Design review of the part built by this model. Coordinates are the model's own, in mm. Face numbers are marked on the shaded views. A direction names the side the tool comes from. Round coordinates to 2 decimals unless told otherwise and drop trailing zeros. Write each loop counter-clockwise with the first axis right and the second up, starting at its lowest first coordinate (ties: lowest second). Pieces come first, ordered by that corner, then holes. Notation, with made-up numbers: M -1.75,37.5 L 53.25,37.5 A20 ccw 53.25,54.5 Z; hole C 40.5,-16 d2. An arc over 180 degrees is marked long. Use CSV: the item, a comma, the result in double quotes.
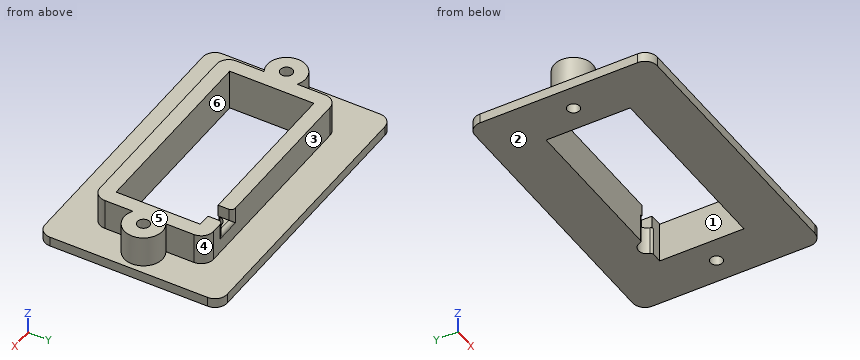
Autodesk Fusion 360 part; units mm, degrees
sketch "Sketch1" plane through (0, 0, 0) normal (0, 0, 1) x (1, 0, 0)
  line L0 (11.6, 5.15) -> (-11.6, 5.15)
  line L1 (-11.6, 5.15) -> (-11.6, -5.15)
  line L2 (-11.6, -5.15) -> (11.6, -5.15)
  line L3 (11.6, -5.15) -> (11.6, 5.15)
  line L4 (11.6, 5.15) -> (-11.6, -5.15) construction
  line L5 (-11.6, 5.15) -> (11.6, -5.15) construction
  line L6 (-17.6, -11.15) -> (17.6, -11.15)
  line L7 (17.6, -11.15) -> (17.6, 11.15)
  line L8 (17.6, 11.15) -> (-17.6, 11.15)
  line L9 (-17.6, 11.15) -> (-17.6, -11.15)
  line L10 (13.4, 6.95) -> (-13.4, 6.95)
  line L11 (-13.4, 6.95) -> (-13.4, -6.95)
  line L12 (-13.4, -6.95) -> (13.4, -6.95)
  line L13 (13.4, -6.95) -> (13.4, 6.95)
  dimension "d1" = 23.2
  dimension "d2" = 10.3
  dimension "d3" = 6
  dimension "d4" = 1.8
extrude "Extrude1" add sketch "Sketch1" along normal blind 7 contours L10 L11 L12 L13
extrude "Extrude2" add sketch "Sketch1" along normal blind 1.2 contours L6 L7 L8 L9
sketch "Sketch2" plane through (0, 0, 0) normal (0, 0, 1) x (1, 0, 0)
  line L0 (-22, 0) -> (23, 0) construction
  circle A0 centre (14.6, 0) radius 0.75 construction
  line L1 (11.6, -5.15) -> (11.6, 5.15) construction
  dimension "d9" = 1.5
  dimension "d10" = 3
sketch "Sketch3" plane through (0, 0, 1.2) normal (0, 0, 1) x (-1, 0, 0)
  line L0 (-13.4, -6.95) -> (-13.4, 6.95)
  line L1 (-13.4, 6.95) -> (13.4, 6.95)
  line L2 (13.4, 6.95) -> (13.4, -6.95)
  line L3 (13.4, -6.95) -> (-13.4, -6.95)
  line L4 (17.6, -11.15) -> (17.6, 11.15)
  line L5 (17.6, 11.15) -> (-17.6, 11.15)
  line L6 (-17.6, 11.15) -> (-17.6, -11.15)
  line L7 (-17.6, -11.15) -> (17.6, -11.15)
  circle A0 centre (-14.6, 0) radius 0.75
  circle A1 centre (-14.6, 0) radius 2.35
  dimension "d11" = 1.6
extrude "Extrude3" add sketch "Sketch3" along normal blind 5 contours L0 A1 picked at (-13.55, 0)
extrude "Extrude9" cut 1 faces at (14.8389, -0.0008, 1.2) along direction (0, 0, -1) up to surface (1.2 mm away)
mirror "Mirror1" about plane through (0, 0, 0) normal (1, 0, 0) of "Extrude2", "Extrude3"
sketch "Sketch4" plane through (0, 0, 0) normal (0, 0, 1) x (1, 0, 0)
  line L0 (11.6, -1) -> (17.6, -1)
  line L1 (17.6, -1) -> (17.6, 0.9)
  line L2 (17.6, 0.9) -> (11.6, 0.9)
  line L3 (11.6, 0.9) -> (11.6, -1)
sketch "Sketch5" plane through (0, 0, 0) normal (0, 0, 1) x (1, 0, 0)
  arc A0 (10.0479, 5.1477) -> (7.9479, 5.146) centre (8.9979, 5.148) ccw
  line L0 (7.9479, 5.146) -> (10.0479, 5.1477)
  dimension "d17" = 1.05
extrude "Extrude4" cut sketch "Sketch5" along normal up to surface (7 mm away)
extrude "Extrude5" add 2 faces at (13.55, 0, 6.2) (-13.55, 0, 6.2) along direction (0, 0, 1) up to surface end surface through (0, 0, 7) normal (0, 0, 1) offset 0
sketch "Sketch6" plane through (0, 0, 7) normal (0, 0, 1) x (-1, 0, 0)
  circle A0 centre (14.6, 0) radius 0.75
  circle A1 centre (-14.6, 0) radius 0.75
  line L0 (-13.4, 6.95) -> (-13.4, 2.0205)
  arc A2 (-13.4, 2.0205) -> (-13.4, -2.0205) centre (-14.6, 0) ccw
  line L1 (-13.4, -2.0205) -> (-13.4, -6.95)
  line L2 (-13.4, -6.95) -> (13.4, -6.95)
  line L3 (13.4, -6.95) -> (13.4, -2.0205)
  arc A3 (13.4, -2.0205) -> (13.4, 2.0205) centre (14.6, 0) ccw
  line L4 (13.4, 2.0205) -> (13.4, 6.95)
  line L5 (13.4, 6.95) -> (-13.4, 6.95)
  arc A4 (-10.0479, -5.15) -> (-7.9479, -5.15) centre (-8.9979, -5.148) ccw
  line L6 (-10.0479, -5.15) -> (-11.6, -5.15)
  line L7 (-11.6, -5.15) -> (-11.6, 5.15)
  line L8 (-11.6, 5.15) -> (11.6, 5.15)
  line L9 (11.6, 5.15) -> (11.6, -5.15)
  line L10 (11.6, -5.15) -> (-7.9479, -5.15)
  line L11 (-10.0479, -5.15) -> (-10.0444, -6.95)
  line L12 (-7.9479, -5.15) -> (-7.9514, -6.95)
extrude "Extrude6" cut sketch "Sketch6" against normal blind 1.5 contours L2 A4 L11 L12
extrude "Extrude7" cut 1 faces at (8.9718, 6.6983, 5.5) along direction (0, 0, -1) blind 2
extrude "Extrude8" cut 1 faces at (-3.8667, -6.35, 7) along direction (0, 0, -1) blind 2
fillet "Fillet1" radius 0.35 2 edges at (7.9479, 5.15, 2.75) (10.0479, 5.15, 2.75)
fillet "Fillet2" radius 1.5 8 edges at (13.4, -6.95, 4.1) (13.4, 6.95, 4.1) (-13.4, -6.95, 4.1) (-13.4, 6.95, 4.1) (17.6, -11.15, 0.6) (-17.6, -11.15, 0.6) (-17.6, 11.15, 0.6) (17.6, 11.15, 0.6)
fillet "Fillet5" radius 0.5 3 edges at (8.9979, 6.95, 3.5) (7.9514, 6.95, 4.25) (10.0444, 6.95, 4.25)
extrude "Extrude10" cut 1 faces at (14.3611, -0.4138, 1.2) along direction (0, 0, -1) blind 2
extrude "Extrude11" cut 1 faces at (-14.4167, 0.2446, 1.2) along direction (0, 0, -1) blind 2
1) Add section A-A on z = 1.9. Write out the cut boundary in (x, y), then the cut area to 3 significant figures.
Answers:
outline,"M -13.4,-5.45 A1.5 ccw -11.9,-6.95 L 11.9,-6.95 A1.5 ccw 13.4,-5.45 L 13.4,-2.02 A2.35 ccw long 13.4,2.02 L 13.4,5.45 A1.5 ccw 11.9,6.95 L -11.9,6.95 A1.5 ccw -13.4,5.45 L -13.4,2.02 A2.35 ccw long -13.4,-2.02 Z; hole C -14.6,0 d1.5; hole M -11.6,-5.15 L 11.6,-5.15 L 11.6,5.15 L 10.35,5.15 A0.35 cw 10.01,5.41 A1.05 ccw 7.98,5.41 A0.35 cw 7.64,5.15 L -11.6,5.15 Z; hole C 14.6,0 d1.5"
area,"154 mm²"
2) Add section B-B on y = 0. Write out the cut boundary in (x, z), then the cut area to 3 significant figures.
Answers:
outline,"M -17.6,0 L -15.35,0 L -15.35,5 L -16.95,5 L -16.95,1.2 L -17.6,1.2 Z; M -13.85,0 L -11.6,0 L -11.6,5 L -13.85,5 Z; M 11.6,0 L 13.85,0 L 13.85,5 L 11.6,5 Z; M 15.35,0 L 17.6,0 L 17.6,1.2 L 16.95,1.2 L 16.95,5 L 15.35,5 Z"
area,"40.1 mm²"
3) Add section C-C on x = -14.6. Write out the cut boundary in (y, z).
Answers:
outline,"M -11.15,0 L -0.75,0 L -0.75,5 L -2.35,5 L -2.35,1.2 L -11.15,1.2 Z; M 0.75,0 L 11.15,0 L 11.15,1.2 L 2.35,1.2 L 2.35,5 L 0.75,5 Z"
4) Wall thickness on line 1 along X through (y, z) = (0, 2.8); line 2 along Y through (x, z) = (-14.6, 3.65); line 3 along X through (y, z) = (5.25, 3.8): over which ranges is each line inside the solid? List them lowest first. Write a range as [from, to].
Answers:
line 1,"[-16.95, -15.35], [-13.85, -11.6], [11.6, 13.85], [15.35, 16.95]"
line 2,"[-2.35, -0.75], [0.75, 2.35]"
line 3,"[-13.4, 7.95], [10.05, 13.4]"
5) The part is to be moulded in two halves that separate along Y. For the marked faces 1, 2 and 3, say which applies: released by +Y, released by -Y, zero draft, split by the parting line, or undercut.
Answers:
face 1,"undercut"
face 2,"zero draft"
face 3,"released by +Y"
6) Add section D-D on z = 4.15. Write out the cut boundary in (x, y).
Answers:
outline,"M -13.4,-5.45 A1.5 ccw -11.9,-6.95 L 11.9,-6.95 A1.5 ccw 13.4,-5.45 L 13.4,-2.02 A2.35 ccw long 13.4,2.02 L 13.4,5.45 A1.5 ccw 11.9,6.95 L 10.55,6.95 A0.5 ccw 10.05,6.45 L 10.05,5.15 L 11.6,5.15 L 11.6,-5.15 L -11.6,-5.15 L -11.6,5.15 L 7.95,5.15 L 7.95,6.45 A0.5 ccw 7.45,6.95 L -11.9,6.95 A1.5 ccw -13.4,5.45 L -13.4,2.02 A2.35 ccw long -13.4,-2.02 Z; hole C -14.6,0 d1.5; hole C 14.6,0 d1.5"
7) For pin 1 Ø0.5 at (x, z) = (11, 2.5) entering from -Y; pin 2 Ø1 at (y, z) = (-5, 3) entering from +X; pin 3 Ø1.9 at (x, z) = (1.5, 3.5) entering from +Y, all flat-tipped, find the tip position at first contact; note any pin that passes through.
Answers:
pin 1,"y = -6.95"
pin 2,"x = 13.4"
pin 3,"y = 6.95"
8) Machinability: for the marked faces 4, 5 and 6, which of the approach directions +Z, -Z, +X, -X, +Y, -Y give a long, thin tool a straight path to every point of the face, cutting with its end or side? Answer none if there is none.
Answers:
face 4,"+Z, +X, +Y"
face 5,"+Z, +X, -X, +Y, -Y"
face 6,"+Z, -Z"
